Check sheet for the modelled part. Datum: model origin and axes. Units: mm. Face numbers are marked on the shaded views. A direction names the side the tool comes from. Round coordinates to 2 decimals unless told otherwise and drop trailing zeros. Order: outer loops, then holes, each group sorted by start corner. A loop starts at its lowest first (then second) coordinate and runs counter-clockwise, first axis right, second up. Notation, with made-up numbers: (71.5, -34.75) -> (117.5, -34.75) arc R26 cw to (117.5, -16.75) -> close; hole circle Ø5 at (-28.5, 48.5). An arc over 180 degrees is marked (long way). Answer in a Markdown table with one row per item.
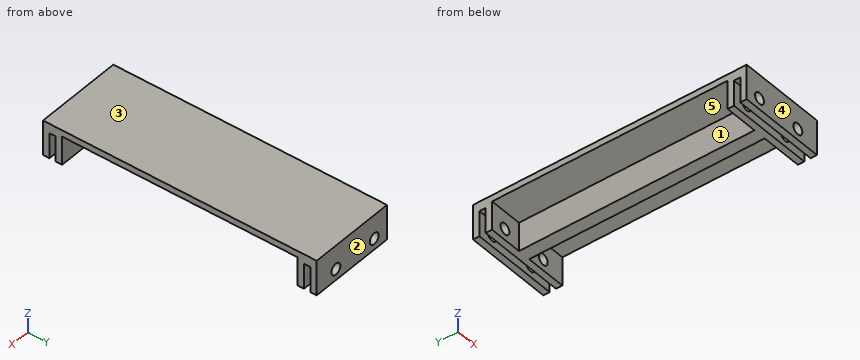
```python
from build123d import *

# Parameters (mm, degrees)
SKETCH_1_W          = 30
SKETCH_1_H          = 11
EXTRUDE_1_DEPTH     = 6
SKETCH_2_W          = 16
SKETCH_2_H          = 2
CUT_EXTRUDE_1_DEPTH = 144
EXTRUDE_2_DEPTH     = 74
SKETCH_4_R          = 1.75
CUT_EXTRUDE_2_DEPTH = 144
SKETCH_5_W          = 11
SKETCH_5_H          = 80
CUT_EXTRUDE_3_DEPTH = 2.5


with BuildPart() as part:
    # 草图1 → 凸台-拉伸1 (new body)
    with BuildSketch(Plane(origin=(0, 0, 0), x_dir=(1, 0, 0), z_dir=(0, 1, 0))):
        Rectangle(SKETCH_1_W, SKETCH_1_H)
    extrude_1 = extrude(amount=EXTRUDE_1_DEPTH)

    # 草图2 → 切除-拉伸1 (cut)
    with BuildSketch(Plane.ZY.offset(15)):
        with Locations((-5.5, 3)):
            Rectangle(SKETCH_2_W, SKETCH_2_H)
    cut_extrude_1 = extrude(amount=-CUT_EXTRUDE_1_DEPTH, mode=Mode.SUBTRACT)

    # 草图3 → 凸台-拉伸2 (add)
    with BuildSketch(Plane(origin=(0, 6, 0), x_dir=(1, 0, 0), z_dir=(0, 1, 0))):
        Polygon((2, 5.5), (-2, 5.5), (-2, -3.5), (-15, -3.5), (-15, -5.5), (15, -5.5), (15, -3.5), (2, -3.5), align=None)
    extrude(amount=EXTRUDE_2_DEPTH)

    # 草图4 → 切除-拉伸2 (cut)
    with BuildSketch(Plane(origin=(0, 6, 0), x_dir=(1, 0, 0), z_dir=(0, 1, 0))):
        with Locations(Location((-7.5, 2, 0), (0, 0, 270))):
            Circle(SKETCH_4_R)
        with Locations(Location((7.5, 2, 0), (0, 0, 270))):
            Circle(SKETCH_4_R)
    cut_extrude_2 = extrude(amount=-CUT_EXTRUDE_2_DEPTH, mode=Mode.SUBTRACT)

    # 草图5 → 切除-拉伸3 (cut)
    with BuildSketch(Plane.ZY.offset(15)):
        with Locations((0, 40)):
            Rectangle(SKETCH_5_W, SKETCH_5_H)
    cut_extrude_3 = extrude(amount=-CUT_EXTRUDE_3_DEPTH, mode=Mode.SUBTRACT)

    # 镜向1: 凸台-拉伸1, 切除-拉伸1, 切除-拉伸2, 切除-拉伸3 across plane
    add(extrude_1.mirror(Plane.ZX.offset(43)))
    add(cut_extrude_1.mirror(Plane.ZX.offset(43)), mode=Mode.SUBTRACT)
    add(cut_extrude_2.mirror(Plane.ZX.offset(43)), mode=Mode.SUBTRACT)
    add(cut_extrude_3.mirror(Plane.ZX.offset(43)), mode=Mode.SUBTRACT)


solid = part.part
```
(1) Draft check along Y on the marked faces 1, 2 and 3. Enter one of: pulls with the +Y half, pulls with the -Y half, needs draft (parallel to the pull), parting line crosses it, or undercut.
Solutions:
| item | result |
|---|---|
| face 1 | undercut |
| face 2 | pulls with the +Y half |
| face 3 | needs draft |
(2) Scan lines: probe 1 along Y at (x, z) = (1.25, -4); probe 2 along Y at (x, z) = (7.5, 0); probe 3 along X at (y, z) = (0.95, -2). Record each from-to range of solid material in increasing order. Write a range as from..to.
Solutions:
| item | result |
|---|---|
| probe 1 | 0..2, 4..82, 84..86 |
| probe 2 | 0..2, 4..6, 80..82, 84..86 |
| probe 3 | -12.5..-9.25, -5.75..5.75, 9.25..15 |
(3) Depth check by flat-ended pin: pin 1 Ø0.6 at (x, y) = (4, 83) entering from -Z. Enter the tip coordinate at first touch or a pass-through.
Solutions:
| item | result |
|---|---|
| pin 1 | z = 2.5 |
(4) Section check B-B on y = 49.5. Record the boundary of the cut face in (x, z), plus the area to 3 significant figures.
Solutions:
| item | result |
|---|---|
| outline | (-12.5, 3.5) -> (-2, 3.5) -> (-2, -5.5) -> (2, -5.5) -> (2, 3.5) -> (15, 3.5) -> (15, 5.5) -> (-12.5, 5.5) -> close |
| area | 91.0 mm^2 |
(5) Tool access check on the marked faces 4 and 5. Record the directions out of +Z, -Z, +X, -X, +Y, -Y that give a thin tool (end or side, any length) a straight path to the whole face; none if there is none.
Solutions:
| item | result |
|---|---|
| face 4 | +Z, -Z, +X, -X, -Y |
| face 5 | -Z, -X |
(6) Section check A-A on x = 7.5. Give the number of separate pieces and of enclosed holes in the cut face, plus the area to 3 significant figures.
Solutions:
| item | result |
|---|---|
| separate pieces | 5 |
| enclosed holes | 0 |
| area | 220 mm^2 |
(7) Section check C-C on x = 3. Record the boundary of the cut face in (y, z).
Solutions:
| item | result |
|---|---|
| outline | (0, -5.5) -> (2, -5.5) -> (2, 2.5) -> (4, 2.5) -> (4, -5.5) -> (6, -5.5) -> (6, 3.5) -> (80, 3.5) -> (80, -5.5) -> (82, -5.5) -> (82, 2.5) -> (84, 2.5) -> (84, -5.5) -> (86, -5.5) -> (86, 5.5) -> (0, 5.5) -> close |
